```python
from build123d import *

# Parameters (mm, degrees)
PAD_DEPTH = 20


with BuildPart() as part:
    # Sketch → Pad (new body)
    with BuildSketch(Plane.XY):
        with BuildLine():
            Line((5.140364, 1.2), (6.594756, 4.907874))
            ThreePointArc((6.594756, 4.907874), (6.142126, 5.944756), (5.105244, 5.492126))
            Line((4.218492, 3.231414), (5.105244, 5.492126))
            Line((4.15, 3.231414), (4.218492, 3.231414))
            Line((4.15, 8.3), (4.15, 3.231414))
            ThreePointArc((4.15, 8.3), (3.915685, 8.865685), (3.35, 9.1))
            Line((0.45, 9.1), (3.35, 9.1))
            ThreePointArc((0.45, 9.1), (-0.115685, 8.865685), (-0.35, 8.3))
            Line((-0.35, 3.199929), (-0.35, 8.3))
            Line((-2.55, 3.199929), (-0.35, 3.199929))
            Line((-2.55, 9.1), (-2.55, 3.199929))
            ThreePointArc((-2.55, 9.1), (-3.35, 9.9), (-4.15, 9.1))
            Line((-4.15, 3.208053), (-4.15, 9.1))
            Line((-4.325596, 3.208053), (-4.15, 3.208053))
            Line((-5.092804, 5.458176), (-4.325596, 3.208053))
            ThreePointArc((-5.092804, 5.458176), (-6.108176, 5.957196), (-6.607196, 4.941824))
            Line((-5.331372, 1.2), (-6.607196, 4.941824))
            Line((-5.331372, 1.2), (0.449979, 1.199852))
            ThreePointArc((0.449979, 1.199852), (1.015678, 1.434159), (1.25, 1.999852))
            Line((1.25, 1.999852), (1.25, 7.009087))
            ThreePointArc((1.740913, 7.5), (1.393785, 7.356215), (1.25, 7.009087))
            Line((1.740913, 7.5), (2.059087, 7.5))
            ThreePointArc((2.55, 7.009087), (2.406215, 7.356215), (2.059087, 7.5))
            Line((2.55, 7.009087), (2.55, 1.99987))
            ThreePointArc((2.55, 1.99987), (2.784335, 1.434164), (3.350058, 1.19987))
            Line((3.350058, 1.19987), (5.140364, 1.2))
        make_face()
    extrude(amount=PAD_DEPTH)


solid = part.part
```
The listing builds one solid part. Answer for the finished solid, in the listing's coordinates (mm). A direction names the side the tool comes from. Round coordinates to 2 decimals unless told otherwise and drop trailing zeros. Write each loop counter-clockwise with the first axis right and the second up, starting at its lowest first coordinate (ties: lowest second). Pieces come first, ordered by that corner, then holes. Notation, with made-up numbers: (82.25, 29) -> (101.25, 29) arc R32 ccw to (101.25, 56) -> close; hole circle Ø10 at (33, 45.25). An arc over 180 degrees is marked (long way). Write item = value, one per line.
1) Section C-C on z = 18.5 is taken. Write down the section's boundary in (x, y).
Check values:
outline = (-6.61, 4.94) -> (-5.33, 1.2) -> (0.45, 1.2) arc R0.8 ccw to (1.25, 2) -> (1.25, 7.01) arc R0.49 cw to (1.74, 7.5) -> (2.06, 7.5) arc R0.49 cw to (2.55, 7.01) -> (2.55, 2) arc R0.8 ccw to (3.35, 1.2) -> (5.14, 1.2) -> (6.59, 4.91) arc R0.8 ccw to (5.11, 5.49) -> (4.22, 3.23) -> (4.15, 3.23) -> (4.15, 8.3) arc R0.8 ccw to (3.35, 9.1) -> (0.45, 9.1) arc R0.8 ccw to (-0.35, 8.3) -> (-0.35, 3.2) -> (-2.55, 3.2) -> (-2.55, 9.1) arc R0.8 ccw to (-4.15, 9.1) -> (-4.15, 3.21) -> (-4.33, 3.21) -> (-5.09, 5.46) arc R0.8 ccw to start
2) Given pin 1 (0.9 mm diameter, centred on x = 2, z = 9.5, fed in from +Y); pin 2 (1 mm diameter, centred on y = 9, z = 9.5, fed in from +X); pin 3 (3 mm diameter, centred on y = 8, z = 7, fed in from -X), each flat-ended and moving along its own axis, determine where each tip first touches the part or whether it passes through.
Check values:
pin_1 = 9.1
pin_2 = 4.12
pin_3 = -4.15
3) Which of the six approach directions +Z, -Z, +X, -X, +Y, -Y give full straight-line access (tool end or side, diameter ignored) to faces 4 (the flat face through (2, 9.1, 10)), 5 (the cylindrical face through (1.01, 1.43, 9.86)), 6 (the flat face through (5.86, 3.03, 9.86)), 7 (the cylindrical face through (-0.11, 8.87, 9.86))?
Check values:
face_4 = +Z, -Z, +X, +Y
face_5 = +Z, -Z, -Y
face_6 = +Z, -Z, +X, -Y
face_7 = +Z, -Z, +Y
4) Section B-B on y = 2.75 is taken. Write down the section's boundary in (x, z).
Check values:
outline = (-5.86, 0) -> (1.25, 0) -> (1.25, 20) -> (-5.86, 20) -> close; (2.55, 0) -> (5.75, 0) -> (5.75, 20) -> (2.55, 20) -> close
5) Section D-D on y = 5.2 is taken. Write down the section's boundary in (x, z).
Check values:
outline = (-6.65, 0) -> (-5, 0) -> (-5, 20) -> (-6.65, 20) -> close; (-4.15, 0) -> (-2.55, 0) -> (-2.55, 20) -> (-4.15, 20) -> close; (-0.35, 0) -> (1.25, 0) -> (1.25, 20) -> (-0.35, 20) -> close; (2.55, 0) -> (4.15, 0) -> (4.15, 20) -> (2.55, 20) -> close; (4.99, 0) -> (6.65, 0) -> (6.65, 20) -> (4.99, 20) -> close
6) For a pull along X with two mould halves and no side action, classify faces 1 (the flat face through (0, 5, 0)), 2 (the flat face through (-0.35, 6, 10)), 3 (the flat face through (-5.96, 3.04, 9.86)) as released by +X, released by -X, zero draft, split by the parting line, or undercut.
Check values:
face_1 = zero draft
face_2 = undercut
face_3 = released by -X
7) Section A-A on y = 6.5 is taken. Write down the section's boundary in (x, z).
Check values:
outline = (-4.15, 0) -> (-2.55, 0) -> (-2.55, 20) -> (-4.15, 20) -> close; (-0.35, 0) -> (1.25, 0) -> (1.25, 20) -> (-0.35, 20) -> close; (2.55, 0) -> (4.15, 0) -> (4.15, 20) -> (2.55, 20) -> close
8) Straight lines are drawn through the part: line 1 along X through (y, z) = (7, 5.25); line 2 along X through (y, z) = (4.25, 11.25); line 3 along X through (y, z) = (4.75, 5). For each, find the intervals that lie inside material, in ascending order. Write a range as [from, to].
Check values:
line_1 = [-4.15, -2.55], [-0.35, 1.25], [2.55, 4.15]
line_2 = [-6.37, -4.68], [-4.15, -2.55], [-0.35, 1.25], [2.55, 4.15], [4.62, 6.34]
line_3 = [-6.54, -4.85], [-4.15, -2.55], [-0.35, 1.25], [2.55, 4.15], [4.81, 6.53]
